Source: CAD feature listing. Evaluate the final solid. Frame: model axes, mm. A direction names the side the tool comes from. Give positions to 0.01 mm unless a question says otherwise; leave off trailing zeros. Order: outer loops, then holes, each group sorted by start corner. A loop starts at its lowest first (then second) coordinate and runs counter-clockwise, first axis right, second up. Notation, with made-up numbers: (13.25, 80) - (44.25, 80) arc R26 cw to (44.25, 112) - close; hole circle Ø2 at (54.25, 27). An arc over 180 degrees is marked (long way). Use CSV: the item, a comma, the result in double quotes.
```python
from build123d import *

# Parameters (mm, degrees)
F0_W      = 90
F0_H      = 42
F1_DEPTH  = 15.3
F2_R      = 20
F3_R      = 20
F4_R      = 13.825
F5_DEPTH  = 7
F6_R      = 5.5
F7_DEPTH  = 10
F8_R      = 7.525
F8_R_2    = 1.2
F9_DEPTH  = 18
F10_R     = 16.825
F10_R_2   = 13.825
F11_DEPTH = 10
F12_SIZE  = 1
F13_SIZE  = 0.5
F14_R     = 2.25
F15_DEPTH = 6


with BuildPart() as f1:
    # F0 (on Top) → F1 (new body)
    with BuildSketch(Plane.XY):
        Rectangle(F0_W, F0_H)
    extrude(amount=F1_DEPTH)

    # F2
    f2_edges = [f1.edges().sort_by_distance(p)[0] for p in [
        (-45, -21, 7.65),
        (-45, 21, 7.65),
    ]]
    fillet(f2_edges, radius=F2_R)

    # F3
    f3_edges = [f1.edges().sort_by_distance(p)[0] for p in [
        (45, 21, 7.65),
        (45, -21, 7.65),
    ]]
    fillet(f3_edges, radius=F3_R)

    # F4 (on face) → F5 (cut)
    with BuildSketch(Plane(origin=(0, 0, 0), x_dir=(1, 0, 0), z_dir=(0, 0, -1))):
        Circle(F4_R)
    extrude(amount=-F5_DEPTH, mode=Mode.SUBTRACT)

    # F6 (on face) → F7 (cut)
    with BuildSketch(Plane.XY.offset(15.3)):
        Circle(F6_R)
    extrude(amount=-F7_DEPTH, mode=Mode.SUBTRACT)

    # F8 (on face) → F9 (cut)
    with BuildSketch(Plane.XY.offset(15.3)):
        with Locations((-30, 0)):
            Circle(F8_R)
        with Locations((30, 0)):
            Circle(F8_R)
        with Locations((-8.15, 0)):
            Circle(F8_R_2)
        with Locations((8.15, 0)):
            Circle(F8_R_2)
    extrude(amount=-F9_DEPTH, mode=Mode.SUBTRACT)

    # F10 (on face) → F11 (join)
    with BuildSketch(Plane(origin=(0, 0, 0), x_dir=(1, 0, 0), z_dir=(0, 0, -1))):
        Circle(F10_R)
        Circle(F10_R_2, mode=Mode.SUBTRACT)
    extrude(amount=F11_DEPTH)

    # F12
    f12_edges = [f1.edges().sort_by_distance(p)[0] for p in [
        (-13.825, 0, -10),
    ]]
    chamfer(f12_edges, length=F12_SIZE)

    # F13
    f13_edges = [f1.edges().sort_by_distance(p)[0] for p in [
        (-37.525, 0, 0),
        (22.475, 0, 0),
    ]]
    chamfer(f13_edges, length=F13_SIZE)

    # F14 (on face) → F15 (cut)
    with BuildSketch(Plane.XY.offset(15.3)):
        with Locations((-8.15, 0)):
            Circle(F14_R)
        with Locations((8.15, 0)):
            Circle(F14_R)
    extrude(amount=-F15_DEPTH, mode=Mode.SUBTRACT)


solid = f1.part
```
Item 1: Section B-B on x = 0. Return the cut outline in (y, z) (3 decimals), then the cut area to 3 significant figures.
Filled in:
outline,"(-21, 0) - (-16.825, 0) - (-16.825, -10) - (-14.825, -10) - (-13.825, -9) - (-13.825, 7) - (-5.5, 7) - (-5.5, 15.3) - (-21, 15.3) - close; (5.5, 7) - (13.825, 7) - (13.825, -9) - (14.825, -10) - (16.825, -10) - (16.825, 0) - (21, 0) - (21, 15.3) - (5.5, 15.3) - close"
area,"417 mm2"
Item 2: Section A-A on z = 12.25. Return the cut outline in (x, y) (3 decimals).
Filled in:
outline,"(-45, -1) arc R20 ccw to (-25, -21) - (25, -21) arc R20 ccw to (45, -1) - (45, 1) arc R20 ccw to (25, 21) - (-25, 21) arc R20 ccw to (-45, 1) - close; hole circle Ø15.05 at (-30, 0); hole circle Ø4.5 at (-8.15, 0); hole circle Ø11 at (0, 0); hole circle Ø4.5 at (8.15, 0); hole circle Ø15.05 at (30, 0)"
Item 3: Section D-D on y = -4.5. Count the separate pieces of the cut face and the enclosed holes in it, then the cut area to 3 significant figures.
Filled in:
separate pieces,"4"
enclosed holes,"0"
area,"824 mm2"
Item 4: First-contact query: pin 1 (1 mm diameter, centred on y = -15, z = -4.5, fed in from +X); pin 2 (1 mm diameter, centred on y = -15, z = 1, fed in from -X); pin 3 (2 mm diameter, centred on x = -8, y = 1, fed in from +Z). Flat tips, straight axial feed; report the tip coordinate or a pass-through.
Filled in:
pin 1,"stops at x = 8.53"
pin 2,"stops at x = -39.76"
pin 3,"stops at z = 9.3"
Item 5: Material intervals for line 1 (X direction, y = 0.5, z = 3.75); line 2 (Y direction, x = -8.15, z = 8.8); line 3 (X direction, y = 3, z = 1.75), sorted ascending. Write a range as from..to.
Filled in:
line 1,"x = -45..-37.51, -22.49..-13.82, 13.82..22.49, 37.51..45"
line 2,"y = -21..-1.2, 1.2..21"
line 3,"x = -44.9..-36.9, -23.1..-13.5, 13.5..23.1, 36.9..44.9"
Item 6: Section C-C on z = -4.25. Return the cut outline in (x, y) (3 decimals), then the cut area to 3 significant figures.
Filled in:
outline,"circle Ø33.65 at (0, 0); hole circle Ø27.65 at (0, 0)"
area,"289 mm2"
Item 7: Set-up query: faces 1 (the flat face through (0, 15, -10)), 2 (the cylindrical face through (5.902, 0.099, 12.342)). Return all of +Z, -Z, +X, -X, +Y, -Y with unobstructed straight access to the full face (end or side cutting, diameter ignored); none if empty.
Filled in:
face 1,"-Z, +X, -X, +Y, -Y"
face 2,"+Z"
Item 8: Mould query, pull axis X, two halves, no side actions, for faces 3 (the flat face through (-7, -1, 9.3)), 4 (the flat face through (0, 21, 8)), 5 (the cylindrical face through (-39.297, 14.986, 7.757)), 6 (the flat face through (0, 6, 7)). Classes: released by +X, released by -X, zero draft, split by the parting line, or undercut.
Filled in:
face 3,"undercut"
face 4,"zero draft"
face 5,"released by -X"
face 6,"undercut"
